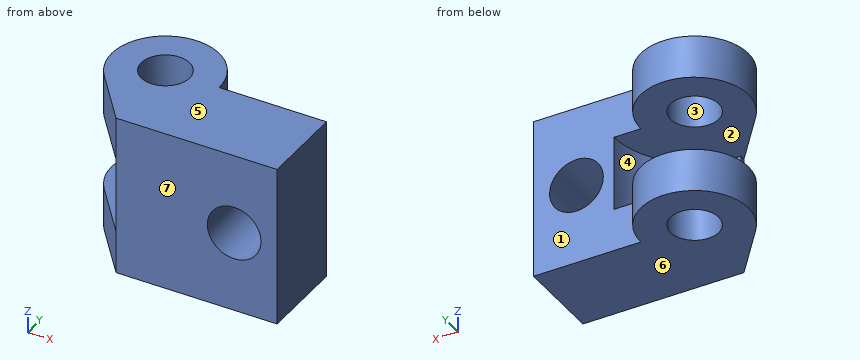
Autodesk Inventor part; units mm, degrees
ref_plane "YZ Plane" through (0, 0, 0) normal (1, 0, 0) x (0, 1, 0)
ref_plane "XZ Plane" through (0, 0, 0) normal (0, 1, 0) x (-1, 0, 0)
ref_plane "XY Plane" through (0, 0, 0) normal (0, 0, 1) x (1, 0, 0)
sketch "Sketch1" plane through (0, 0, 0) normal (0, 1, 0) x (-1, 0, 0)
  line L0 (7.5, 7.5) -> (-7.5, 7.5)
  line L1 (-7.5, 7.5) -> (-7.5, -7.5)
  line L2 (-7.5, -7.5) -> (7.5, -7.5)
  line L3 (7.5, -7.5) -> (7.5, 7.5)
  line L4 (7.5, 7.5) -> (-7.5, -7.5) construction
  line L5 (-7.5, 7.5) -> (7.5, -7.5) construction
  point P0 (0, 0)
  dimension "d0" = 15
  dimension "d1" = 15
extrude "Extrusion1" add sketch "Sketch1" along normal blind 8
sketch "Sketch2" plane through (-7.5, 0, 7.5) normal (0, 0, 1) x (1, 0, 0)
  line L0 (0, 8) -> (15, 8)
  arc A0 (5, 8) -> (-3.9031, 4.875) centre (0, 8) ccw
  line L1 (0, 0) -> (-3.9031, 4.875)
  line L2 (0, 0) -> (0, 8)
  point P0 (7.5, 0)
  dimension "d4" = 10
extrude "Extrusion2" add sketch "Sketch2" against normal blind 4
mirror "Mirror1" about plane through (0, 0, 0) normal (0, 0, 1) of "Extrusion2"
sketch "Sketch3" plane through (-7.5, 0, 3.5) normal (0, 0, -1) x (-1, 0, 0)
  arc A0 (3.9031, 4.875) -> (-5, 8) centre (0, 8) ccw
  circle A1 centre (0, 8) radius 7.5
  point P0 (-7.5, 0)
  dimension "d7" = 15
extrude "Extrusion3" cut sketch "Sketch3" along normal up to surface (7 mm away)
sketch "Sketch4" plane through (7.5, 0, 7.5) normal (0, 0, 1) x (1, 0, 0)
  arc A0 (-10, 8) -> (-18.9031, 4.875) centre (-15, 8) ccw
  point P0 (-7.5, 0)
hole "Hole1" at (-7.5, 8, 7.5) direction (0, 0, -1) diameter 4.5 end through all
sketch "Sketch5" plane through (0, 8, 0) normal (0, 1, 0) x (1, 0, 0)
  line L0 (7.5, -7.5) -> (7.5, 7.5)
  point P0 (0, 0)
  point P1 (3.5, 0)
  dimension "d17" = 4
hole "Hole2" at (3.5, 8, 0) direction (0, -1, 0) diameter 5 end through all
properties part number "Piston Wall Guide Small" material "ABS Plastic"
Check sheet for the modelled part. Datum: model origin and axes. Units: mm. Face numbers are marked on the shaded views. A direction names the side the tool comes from. Give positions to 0.01 mm unless a question says otherwise; leave off trailing zeros. Write each loop counter-clockwise with the first axis right and the second up, starting at its lowest first coordinate (ties: lowest second). Pieces come first, ordered by that corner, then holes.
Item 1: Cross-section at C-C (x = 3.5). Enter the section's corners in (y, z), and give its area (3 significant figures).
Item 2: Scan lines: L1, parallel to Z at x = -3.25, y = 9; L2, parallel to Z at x = 3.5, y = 6.25; L3, parallel to Y at x = 4.25, z = -5.75. Record each from-to range of solid material in increasing order.
Item 3: Draft check along Z on the marked faces 4, 5, 6 and 7. Enter one of: released by +Z, released by -Z, zero draft, split by the parting line, or undercut.
Item 4: Cross-section at A-A (z = -1.5). Enter the section's corners in (x, y).
Item 5: Cross-section at B-B (y = 12). Enter the section's corners in (x, z).
Item 6: Cross-section at D-D (y = 7.5). Enter the section's corners in (x, z), and give its area (3 significant figures).
Item 7: Gauge pin test, flat ends, axial feed: pin 1 (0.6 mm diameter, centred on y = 0, z = 0, fed in from -X); pin 2 (6 mm diameter, centred on x = 3.5, z = 0, fed in from +Y); pin 3 (8 mm diameter, centred on x = 0, z = -3.5, fed in from +Y); pin 4 (8 mm diameter, centred on x = 2, z = 5, fed in from -Y). Record the tip position at first contact, or that the pin passes through.
Item 8: Access from +Z, -Z, +X, -X, +Y, -Y to the whole of each face (thin tool, end or side, straight path). Record for the marked faces 1, 2 and 3.
Report:
1. outline: (0, -7.5) - (8, -7.5) - (8, -2.5) - (0, -2.5) - close; (0, 2.5) - (8, 2.5) - (8, 7.5) - (0, 7.5) - close
1. area: 80.0 mm2
2. L1: z = -7.5 to -3.5, 3.5 to 7.5
2. L2: z = -7.5 to -2.5, 2.5 to 7.5
2. L3: y = 0 to 8
3. face 4: undercut
3. face 5: released by +Z
3. face 6: released by -Z
3. face 7: zero draft
4. outline: (-7.5, 0) - (1.5, 0) - (1.5, 8) - (0, 8) arc R7.5 cw to (-7.5, 0.5) - close; (5.5, 0) - (7.5, 0) - (7.5, 8) - (5.5, 8) - close
5. outline: (-10.5, -7.5) - (-4.5, -7.5) - (-4.5, -3.5) - (-10.5, -3.5) - close; (-10.5, 3.5) - (-4.5, 3.5) - (-4.5, 7.5) - (-10.5, 7.5) - close
6. outline: (-12.47, -7.5) - (-9.69, -7.5) - (-9.69, -3.5) - (-12.47, -3.5) - close; (-12.47, 3.5) - (-9.69, 3.5) - (-9.69, 7.5) - (-12.47, 7.5) - close; (-5.31, -7.5) - (7.5, -7.5) - (7.5, 7.5) - (-5.31, 7.5) - (-5.31, 3.5) - (-0.02, 3.5) - (-0.02, -3.5) - (-5.31, -3.5) - close; hole circle Ø5 at (3.5, 0)
6. area: 158 mm2
7. pin 1: stops at x = -7.5
7. pin 2: stops at y = 8
7. pin 3: stops at y = 11.57
7. pin 4: stops at y = 0
8. face 1: +Z, -Z, +X, +Y
8. face 2: -X, +Y
8. face 3: +Z, -Z
